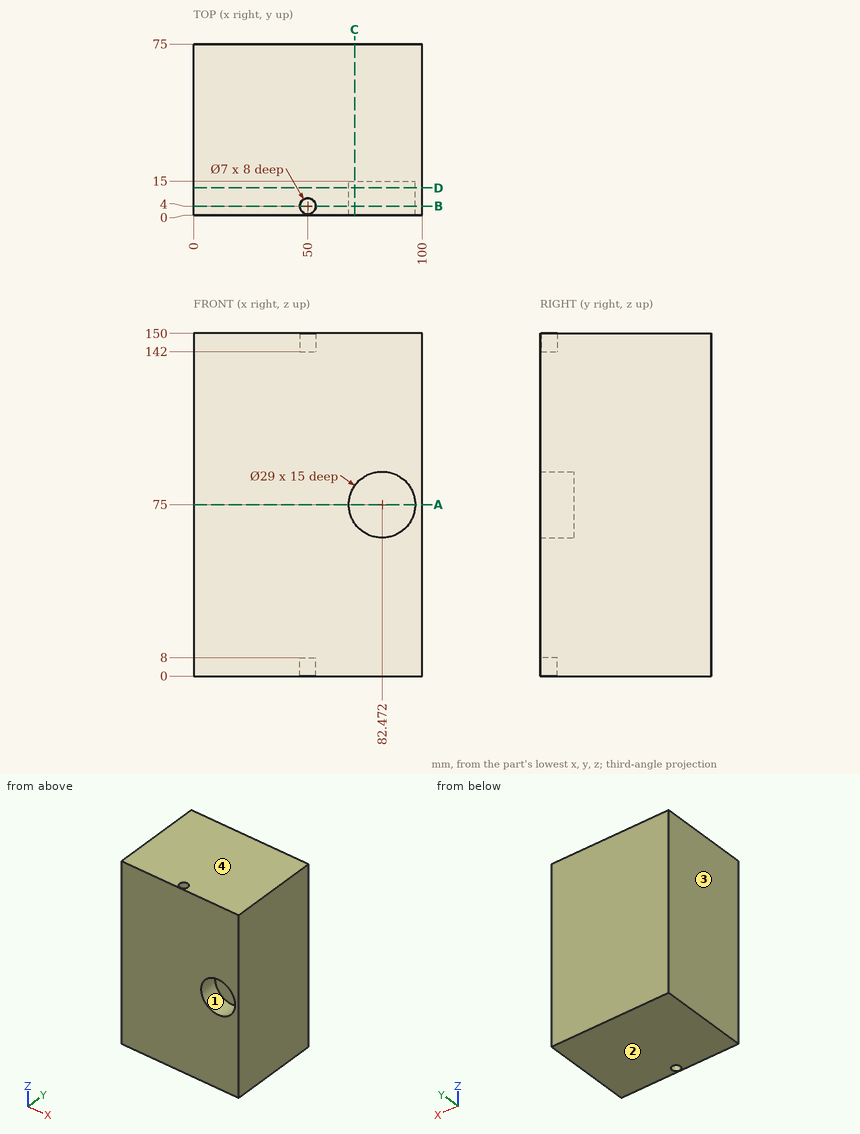
Geometry: see drawing. Coordinates: mm, zero at the bounding-box minimum. Coordinates: 2 decimals unless noted, no trailing zeros. Loops run counter-clockwise (first coordinate to the right, second up) from the corner with the lowest first, then second, coordinate; pieces in that order, holes last. Notation, with made-up numbers: (-26.75, 71.25) -> (-2.75, 71.25) arc R22 cw to (-2.75, 108.25) -> close; hole circle Ø8 at (-19, -16). An arc over 180 degrees is marked (long way). Use a Markdown table: item, result.
1) Pull-direction query (Z, two-part tool) for the marked faces 1, 2, 3 and 4; classes: released by +Z, released by -Z, zero draft, split by the parting line, or undercut.
Results found:
| item | result |
|---|---|
| face 1 | undercut |
| face 2 | released by -Z |
| face 3 | zero draft |
| face 4 | released by +Z |
2) Cut plane A-A (z = 75). Return the cut outline in (x, y), then the cut area to 4 significant figures.
Results found:
| item | result |
|---|---|
| outline | (0, 0) -> (67.97, 0) -> (67.97, 15) -> (96.97, 15) -> (96.97, 0) -> (100, 0) -> (100, 75) -> (0, 75) -> close |
| area | 7,065 mm2 |
3) Material intervals for line 1 along X through (y, z) = (9, 75); line 2 along X through (y, z) = (4, 5); line 3 along Y through (x, z) = (50, 144), sorted ascending. Write a range as from..to.
Results found:
| item | result |
|---|---|
| line 1 | x = 0..67.97, 96.97..100 |
| line 2 | x = 0..46.5, 53.5..100 |
| line 3 | y = 0..0.5, 7.5..75 |
4) Contact query for flat-ended pins moving along their axis: pin 1 (3.5 mm diameter, centred on x = 49, y = 5, fed in from -Z); pin 2 (23 mm diameter, centred on x = 82.47, z = 75, fed in from -Y); pin 3 (1 mm diameter, centred on x = 21, z = 97.5, fed in from -Y); pin 4 (3.5 mm diameter, centred on x = 48.5, y = 4.5, fed in from +Z). Output: stop coordinate, or through.
Results found:
| item | result |
|---|---|
| pin 1 | stops at z = 8 |
| pin 2 | stops at y = 15 |
| pin 3 | stops at y = 0 |
| pin 4 | stops at z = 142 |
5) Cut plane C-C (x = 70.5). Return the cut outline in (y, z), then the cut area to 3 significant figures.
Results found:
| item | result |
|---|---|
| outline | (0, 0) -> (75, 0) -> (75, 150) -> (0, 150) -> (0, 83.18) -> (15, 83.18) -> (15, 66.82) -> (0, 66.82) -> close |
| area | 11,000 mm2 |
6) Cut plane D-D (y = 12). Return the cut outline in (x, z).
Results found:
| item | result |
|---|---|
| outline | (0, 0) -> (100, 0) -> (100, 150) -> (0, 150) -> close; hole circle Ø29 at (82.47, 75) |
7) Cut plane B-B (y = 4). Return the cut outline in (x, z), then the cut area to 3 significant figures.
Results found:
| item | result |
|---|---|
| outline | (0, 0) -> (46.5, 0) -> (46.5, 8) -> (53.5, 8) -> (53.5, 0) -> (100, 0) -> (100, 150) -> (53.5, 150) -> (53.5, 142) -> (46.5, 142) -> (46.5, 150) -> (0, 150) -> close; hole circle Ø29 at (82.47, 75) |
| area | 14,200 mm2 |
